Could you check a few things on this model? Use its own coordinates, in mm. Face numbers are marked on the shaded views. A direction names the side the tool comes from. Give positions to 0.01 mm unless a question says otherwise; leave off trailing zeros. Write each loop counter-clockwise with the first axis right and the second up, starting at its lowest first coordinate (ties: lowest second). Pieces come first, ordered by that corner, then holes. Notation, with made-up numbers: (26, 69.5) - (65, 69.5) arc R16 cw to (65, 94.5) - close; hole circle Ø6 at (-36, 29). An arc over 180 degrees is marked (long way). Write item = value, one per line.
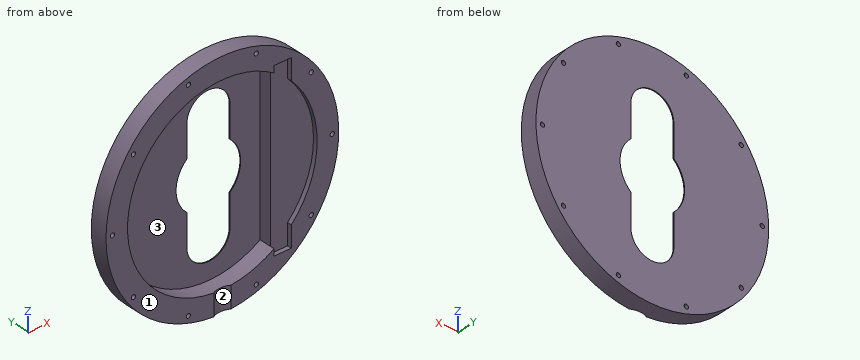
Autodesk Inventor part; units mm, degrees
ref_plane "YZ Plane" through (0, 0, 0) normal (1, 0, 0) x (0, 1, 0)
ref_plane "XZ Plane" through (0, 0, 0) normal (0, 1, 0) x (-1, 0, 0)
ref_plane "XY Plane" through (0, 0, 0) normal (0, 0, 1) x (1, 0, 0)
sketch "Sketch1" plane through (0, 0, 0) normal (0, 1, 0) x (-1, 0, 0)
  circle A0 centre (0, 0) radius 135
  circle A1 centre (0, 0) radius 110
  dimension "d0" = 270
  dimension "d1" = 220
extrude "Extrusion1" add sketch "Sketch1" along normal blind 55
sketch "Sketch2" plane through (0, 0, 0) normal (0, 0, 1) x (1, 0, 0)
  circle A0 centre (0, 5) radius 18
  line L0 (135, 0) -> (-135, 0)
  point P0 (0, 0)
  dimension "d4" = 36
  dimension "d5" = 5
extrude "Extrusion2" cut sketch "Sketch2" against normal through all
sketch "Sketch3" plane through (0, 0, 0) normal (0, -1, 0) x (1, 0, 0)
  circle A0 centre (0, 0) radius 140
extrude "Extrusion3" cut sketch "Sketch3" against normal blind 20
sketch "Sketch4" plane through (0, 20, 0) normal (0, -1, 0) x (1, 0, 0)
  line L0 (0, 0) -> (70, 0)
  line L1 (80, -100) -> (60, -100)
  line L2 (60, -100) -> (60, 100)
  line L3 (60, 100) -> (80, 100)
  line L4 (80, 100) -> (80, -100)
  line L5 (80, -100) -> (60, 100) construction
  line L6 (60, -100) -> (80, 100) construction
  dimension "d10" = 70
  dimension "d11" = 20
  dimension "d12" = 200
extrude "Extrusion4" cut sketch "Sketch4" against normal through all
sketch "Sketch5" plane through (0, 55, 0) normal (0, 1, 0) x (1, 0, 0)
  circle A0 centre (0, 0) radius 127.5
  circle A1 centre (127.5, 0) radius 2
  circle A2 centre (103.1497, 74.9426) radius 2
  circle A3 centre (39.3997, 121.2597) radius 2
  circle A4 centre (-39.3997, 121.2597) radius 2
  circle A5 centre (-103.1497, 74.9426) radius 2
  circle A6 centre (-127.5, 0) radius 2
  circle A7 centre (-103.1497, -74.9426) radius 2
  circle A8 centre (-39.3997, -121.2597) radius 2
  circle A9 centre (39.3997, -121.2597) radius 2
  circle A10 centre (103.1497, -74.9426) radius 2
  dimension "d15" = 255
  dimension "d16" = 4
  dimension "d19" = 360
hole "Hole1" at (127.5, 55, 0) at (103.1497, 55, 74.9426) at (39.3997, 55, 121.2597) at (-39.3997, 55, 121.2597) at (-103.1497, 55, 74.9426) at (-127.5, 55, 0) at (-103.1497, 55, -74.9426) at (-39.3997, 55, -121.2597) at (39.3997, 55, -121.2597) at (103.1497, 55, -74.9426) direction (0, -1, 0) diameter 5 end through all
sketch "Sketch6" plane through (0, 55, 0) normal (0, 1, 0) x (1, 0, 0)
  circle A0 centre (0, 0) radius 140
extrude "Extrusion5" cut sketch "Sketch6" against normal blind 15
sketch "Sketch7" plane through (0, 40, 0) normal (0, 1, 0) x (1, 0, 0)
  circle A0 centre (0, 0) radius 140
  line L0 (80, -100) -> (80, -75.4983)
  line L1 (80, -100) -> (80, -75.4983)
  line L2 (60, -100) -> (80, -100)
  line L3 (80, -100) -> (60, -100)
  line L4 (60, -100) -> (60, -92.1954)
  line L5 (60, 100) -> (60, 92.1954)
  line L6 (60, 92.1954) -> (60, 100)
  line L7 (60, 100) -> (80, 100)
  line L8 (80, 100) -> (80, 75.4983)
  arc A1 (80, -75.4983) -> (80, 75.4983) centre (0, 0) ccw
  arc A2 (60, 92.1954) -> (60, -92.1954) centre (0, 0) ccw
  arc A3 (-25, -65) -> (25, -65) centre (0, -65) ccw
  arc A4 (25, 65) -> (-25, 65) centre (0, 65) ccw
  arc A5 (25, -27.9508) -> (25, 27.9508) centre (0, 0) ccw
  arc A6 (-25, 27.9508) -> (-25, -27.9508) centre (0, 0) ccw
  line L9 (25, 65) -> (25, 27.9508)
  line L10 (25, -27.9508) -> (25, -65)
  line L11 (-25, -65) -> (-25, -27.9508)
  line L12 (-25, 27.9508) -> (-25, 65)
extrude "Extrusion6" add sketch "Sketch7" against normal blind 1 contours L2 L4 A2 L5 L7 L8 A1 L0
sketch "Sketch8" plane through (0, 39, 0) normal (0, -1, 0) x (1, 0, 0)
  line L0 (80, -75.4983) -> (80, -100)
  line L1 (80, -100) -> (60, -100)
  line L2 (60, -100) -> (60, 100)
  line L3 (60, 100) -> (80, 100)
  line L4 (80, 100) -> (80, 75.4983)
  line L5 (80, -75.4983) -> (80, -100)
  arc A0 (80, -75.4983) -> (80, 75.4983) centre (0, 0) ccw
  arc A1 (60, 92.1954) -> (60, -92.1954) centre (0, 0) ccw
extrude "Extrusion7" add sketch "Sketch8" along normal blind 14 contours L0 L1 L2 L3 L4 A0
properties part number "Cylinder Spacer Top"
1. For pin 1 (2.5 mm diameter, centred on x = 71, y = 21.5, fed in from -Z); pin 2 (1.1 mm diameter, centred on y = 39.5, z = -39, fed in from +X); pin 3 (4 mm diameter, centred on y = 23, z = -94, fed in from +X); pin 4 (3 mm diameter, centred on x = -127.5, z = 0, fed in from +Y), each with a flat end and sliding along its axis, tell me the tip position at first contact or that it passes through.
Filled sheet:
pin_1 = -115.59
pin_2 = 129.41
pin_3 = 98.8
pin_4 = through
2. If we section it at D-D, the plane x = -72: Please give me the cut outline in (y, z).
Filled sheet:
outline = (20, -114.2) - (40, -114.2) - (40, 114.2) - (20, 114.2) - (20, 83.16) - (39, 83.16) - (39, -83.16) - (20, -83.16) - close
3. Which directions (+Z, -Z, +X, -X, +Y, -Y) give clear straight access to the entire face, cutting with the end or side of a thin tool? Please do the marked faces 1, 2 and 3.
Filled sheet:
face_1 = +Z, -Z, +X, -X, -Y
face_2 = -Z, -Y
face_3 = -Y
4. If we section it at C-C, the plane y = 29.75: Count the separate pieces of the cut face and the enclosed holes in it, and give its area (3 significant figures).
Filled sheet:
separate_pieces = 1
enclosed_holes = 11
area = 25,500 mm2
5. If we section it at A-A, the plane x = 0: Please give me the cut outline in (y, z).
Filled sheet:
outline = (20, 110) - (39, 110) - (39, 90) - (40, 90) - (40, 135) - (20, 135) - close; (23, -135) - (40, -135) - (40, -90) - (39, -90) - (39, -110) - (23, -110) - close
6. If we section it at B-B, the plane z = 33: Please give me the cut outline in (x, y), and give its area (3 significant figures).
Filled sheet:
outline = (-130.9, 20) - (-104.93, 20) - (-104.93, 39) - (-25, 39) - (-25, 40) - (-130.9, 40) - close; (25, 39) - (60, 39) - (60, 25) - (104.93, 25) - (104.93, 20) - (130.9, 20) - (130.9, 40) - (25, 40) - close
area = 1,830 mm2
7. I need wall thicknesses on line 1 (X direction, y = 35, z = 0); line 2 (Y direction, x = 42.5, z = 35); line 3 (Z direction, x = 0, y = 30). Which ranges of each line are inside material? Lowest first, please.
Filled sheet:
line_1 = -135 to -130, -125 to -110, 60 to 125, 130 to 135
line_2 = 39 to 40
line_3 = -135 to -110, 110 to 135
